Verification items for this drawing (mm, ordinates from the low corner). Coordinates: 2 decimals unless noted, no trailing zeros. Order: outer loops, then holes, each group sorted by start corner. A loop starts at its lowest first (then second) coordinate and runs counter-clockwise, first axis right, second up. Notation, with made-up numbers: (60.5, 75.5) -> (70.5, 75.5) arc R7 cw to (70.5, 84.5) -> close; hole circle Ø10 at (19, 76). An arc over 180 degrees is marked (long way). Write item = value, one per line. Start each with the question number.
1. Cross-section at B-B on z = 69.85. Record the cut outline in (x, y).
2. Go/stop test with flat-tipped pins: P1, Ø0.8, axis at x = 8.5, y = 0.5, coming from the +Z side; P2, Ø0.8, axis at y = 1, z = 54.5, coming from the -X side. Record where each tip stops, or that it passes through.
3. Thickness scan on line 1 along Z through (x, y) = (31.75, 1.2); line 2 along Z through (x, y) = (6.35, 1.25); line 3 along X through (y, z) = (1.05, 19). Record the ranges inside material, lowest first. Write a range as from..to.
4. Cross-section at D-D on z = 57.15. Record the cut outline in (x, y).
5. Cross-section at A-A on x = 31.75. Record the cut outline in (y, z).
6. Cross-section at C-C on x = 57.15. Record the cut outline in (y, z).
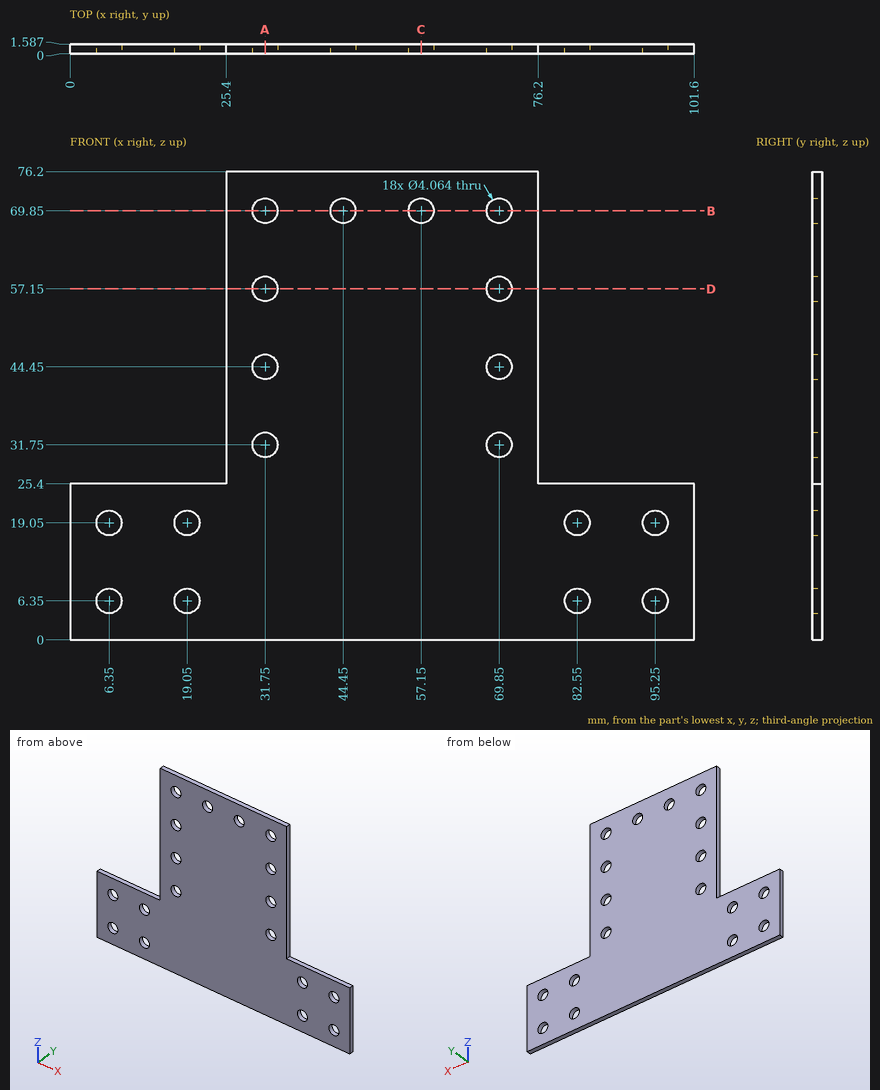
Worked out:
q1.outline = (25.4, 0) -> (29.72, 0) -> (29.72, 1.59) -> (25.4, 1.59) -> close; (33.78, 0) -> (42.42, 0) -> (42.42, 1.59) -> (33.78, 1.59) -> close; (46.48, 0) -> (55.12, 0) -> (55.12, 1.59) -> (46.48, 1.59) -> close; (59.18, 0) -> (67.82, 0) -> (67.82, 1.59) -> (59.18, 1.59) -> close; (71.88, 0) -> (76.2, 0) -> (76.2, 1.59) -> (71.88, 1.59) -> close
q2.P1 = 25.4
q2.P2 = 25.4
q3.line_1 = 0..29.72, 33.78..42.42, 46.48..55.12, 59.18..67.82, 71.88..76.2
q3.line_2 = 0..4.32, 8.38..17.02, 21.08..25.4
q3.line_3 = 0..4.32, 8.38..17.02, 21.08..80.52, 84.58..93.22, 97.28..101.6
q4.outline = (25.4, 0) -> (29.72, 0) -> (29.72, 1.59) -> (25.4, 1.59) -> close; (33.78, 0) -> (67.82, 0) -> (67.82, 1.59) -> (33.78, 1.59) -> close; (71.88, 0) -> (76.2, 0) -> (76.2, 1.59) -> (71.88, 1.59) -> close
q5.outline = (0, 0) -> (1.59, 0) -> (1.59, 29.72) -> (0, 29.72) -> close; (0, 33.78) -> (1.59, 33.78) -> (1.59, 42.42) -> (0, 42.42) -> close; (0, 46.48) -> (1.59, 46.48) -> (1.59, 55.12) -> (0, 55.12) -> close; (0, 59.18) -> (1.59, 59.18) -> (1.59, 67.82) -> (0, 67.82) -> close; (0, 71.88) -> (1.59, 71.88) -> (1.59, 76.2) -> (0, 76.2) -> close
q6.outline = (0, 0) -> (1.59, 0) -> (1.59, 67.82) -> (0, 67.82) -> close; (0, 71.88) -> (1.59, 71.88) -> (1.59, 76.2) -> (0, 76.2) -> close
